Geometry check sheet. Reference: the model listing, model coordinates, mm. Face numbers are marked on the shaded views. A direction names the side the tool comes from. Give positions to 0.01 mm unless a question says otherwise; leave off trailing zeros. Write each loop counter-clockwise with the first axis right and the second up, starting at its lowest first coordinate (ties: lowest second). Pieces come first, ordered by that corner, then holes.
(1) Thickness scan on line 1 along X through (y, z) = (0.75, -12.7); line 2 along Y through (x, z) = (44.45, -23.55); line 3 along Z through (x, y) = (12.7, 2). Record the ranges inside material, lowest first.
(2) Tool access check on the marked faces 1 and 2. Record the directions out of +Z, -Z, +X, -X, +Y, -Y that give a thin tool (end or side, any length) a straight path to the whole face; none if there is none.
(3) Cross-section at D-D (z = -23.5). Record the boundary of the cut face in (x, y).
(4) Cross-section at B-B (x = 38.1). Record the boundary of the cut face in (y, z) (3 decimals), and give its area (3 significant figures).
(5) Cross-section at C-C (z = -12.7). Record the boundary of the cut face in (x, y) (3 decimals), and give its area (3 significant figures).
(6) Cross-section at A-A (x = 25.4). Record the boundary of the cut face in (y, z) (3 decimals).
(7) Mould release check, pull along Y, two halves, no side actions. Record for the marked faces 3, 4, 5 and 6: +Y half, -Y half, draft (parallel to the pull), parting line (faces both ways), or undercut.
(8) Depth check by flat-ended pin: P1, Ø6, axis at x = 28.5, y = 9, coming from the +Z side (3 decimals); P2, Ø11, axis at x = 25, z = -14, coming from the +Y side (3 decimals). Enter the tip coordinate at first touch or a pass-through.
Autodesk Inventor part; units mm, degrees
ref_plane "YZ Plane" through (0, 0, 0) normal (1, 0, 0) x (0, 1, 0)
ref_plane "XZ Plane" through (0, 0, 0) normal (0, 1, 0) x (-1, 0, 0)
ref_plane "XY Plane" through (0, 0, 0) normal (0, 0, 1) x (1, 0, 0)
sketch "Sketch1" plane through (0, 0, 0) normal (1, 0, 0) x (0, 1, 0)
  line L0 (0, 0) -> (3.175, 0)
  line L1 (3.175, 0) -> (3.175, -22.225)
  line L2 (3.175, -25.4) -> (0, -25.4)
  line L3 (0, -25.4) -> (0, 0)
  line L4 (3.175, -25.4) -> (25.4, -25.4)
  line L5 (25.4, -25.4) -> (25.4, -22.225)
  line L6 (25.4, -22.225) -> (3.175, -22.225)
  line L7 (3.175, -22.225) -> (3.175, -25.4)
  dimension "d0" = 3.175
  dimension "d1" = 25.4
  dimension "d2" = 22.225
  dimension "d3" = 3.175
extrude "Extrusion1" add sketch "Sketch1" along normal blind 50.8
sketch "Sketch2" plane through (0, 3.175, 0) normal (0, 1, 0) x (1, 0, 0)
  line L0 (0, 0) -> (0, 25.4) construction
  line L1 (0, 12.7) -> (12.7, 12.7) construction
  line L2 (12.7, 12.7) -> (12.7, 0) construction
  line L3 (0, 0) -> (50.8, 0) construction
  line L4 (25.4, 12.7) -> (38.1, 12.7) construction
  circle A0 centre (12.7, 12.7) radius 2.5797
  circle A1 centre (25.4, 12.7) radius 2.5797
  circle A2 centre (38.1, 12.7) radius 2.5797
  dimension "d6" = 12.7
  dimension "d7" = 12.7
  dimension "d8" = 5.1594
  dimension "d9" = 5.1594
  dimension "d10" = 5.1594
extrude "Extrusion2" cut sketch "Sketch2" against normal blind 50.8
sketch "Sketch3" plane through (0, 3.175, -22.225) normal (0, 0, 1) x (1, 0, 0)
  line L0 (0, 22.225) -> (0, 0) construction
  line L1 (50.8, 22.225) -> (50.8, 0) construction
  line L2 (0, 22.225) -> (50.8, 22.225) construction
  line L3 (25.4, 22.225) -> (25.4, 9.525) construction
  line L4 (25.4, 9.525) -> (44.45, 9.525) construction
  line L5 (25.4, 9.525) -> (6.35, 9.525) construction
  circle A0 centre (25.4, 9.525) radius 2.5797
  circle A1 centre (44.45, 9.525) radius 2.5797
  circle A2 centre (6.35, 9.525) radius 2.5797
  point P0 (0, -3.175)
  dimension "d22" = 12.7
  dimension "d23" = 19.05
  dimension "d24" = 19.05
  dimension "d25" = 5.1594
  dimension "d26" = 5.1594
  dimension "d27" = 5.1594
extrude "Extrusion3" cut sketch "Sketch3" against normal blind 50.8
properties part number "ball gripper to hatch attachment"
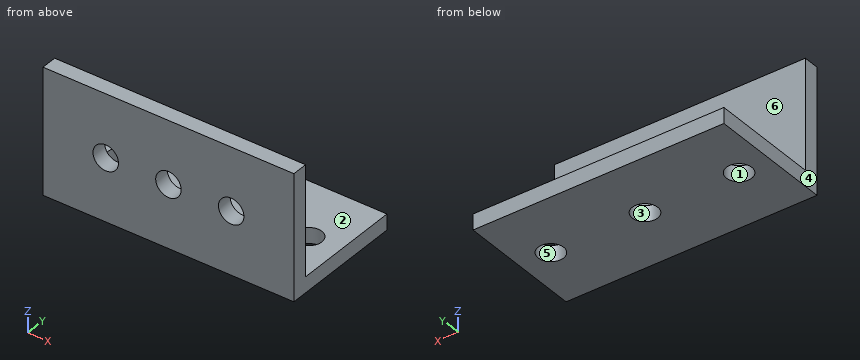
Reply:
1. line 1: x = 0 to 10.12, 15.28 to 22.82, 27.98 to 35.52, 40.68 to 50.8
1. line 2: y = 0 to 10.12, 15.28 to 25.4
1. line 3: z = -25.4 to -15.28, -10.12 to 0
2. face 1: +Z, -Z
2. face 2: +Z, +X, -X, +Y
3. outline: (0, 0) - (50.8, 0) - (50.8, 25.4) - (0, 25.4) - close; hole circle Ø5.16 at (6.35, 12.7); hole circle Ø5.16 at (25.4, 12.7); hole circle Ø5.16 at (44.45, 12.7)
4. outline: (0, -25.4) - (25.4, -25.4) - (25.4, -22.225) - (3.175, -22.225) - (3.175, -15.28) - (0, -15.28) - close; (0, -10.12) - (3.175, -10.12) - (3.175, 0) - (0, 0) - close
4. area: 135 mm2
5. outline: (0, 0) - (10.12, 0) - (10.12, 3.175) - (0, 3.175) - close; (15.28, 0) - (22.82, 0) - (22.82, 3.175) - (15.28, 3.175) - close; (27.98, 0) - (35.52, 0) - (35.52, 3.175) - (27.98, 3.175) - close; (40.68, 0) - (50.8, 0) - (50.8, 3.175) - (40.68, 3.175) - close
5. area: 112 mm2
6. outline: (0, -25.4) - (10.12, -25.4) - (10.12, -22.225) - (3.175, -22.225) - (3.175, -15.28) - (0, -15.28) - close; (0, -10.12) - (3.175, -10.12) - (3.175, 0) - (0, 0) - close; (15.28, -25.4) - (25.4, -25.4) - (25.4, -22.225) - (15.28, -22.225) - close
7. face 3: undercut
7. face 4: draft
7. face 5: undercut
7. face 6: +Y half
8. P1: stops at z = -22.225
8. P2: stops at y = 3.175
